Geometry: final body of the model. Coordinates: model frame, mm. A direction names the side the tool comes from. Round coordinates to 2 decimals unless told otherwise and drop trailing zeros. Write each loop counter-clockwise with the first axis right and the second up, starting at its lowest first coordinate (ties: lowest second). Pieces come first, ordered by that corner, then holes. Notation, with made-up numbers: M 12.25,-4.5 L 21.25,-4.5 A15 ccw 21.25,0.5 Z; hole C 75,8.25 d1. An arc over 180 degrees is marked long. Answer as CSV lines item,"result". Start each with the question number.
Q1. Section query B-B on y = 0. Output: boundary loops of the cut face in (x, z).
Q2. Reachability of faces 1 (the flat face through (-1, 1, -7.914)), 2 (the flat face through (12, 28.5, -3.914)) from +Z, -Z, +X, -X, +Y, -Y: full face, straight path, thin tool, end or side. Return the list, or none.
Q3. Ray query, probe 1 along Y at (x, z) = (7, 17); probe 2 along Z at (x, y) = (31, -8); probe 3 along Z at (x, y) = (9, -32). Return the intervals inside material, ascending.
Q4. First-contact query: pin 1 (3 mm diameter, centred on x = 13.5, y = -9, fed in from +Z); pin 2 (1 mm diameter, centred on y = -5, z = 25, fed in from -X). Flat tips, straight axial feed; report the tip coordinate or a pass-through.
Q5. Mould query, pull axis Y, two halves, no side actions, for faces 3 (the cylindrical face through (-1.18, -36.836, -7.407)), 4 (the cylindrical face through (3.503, 0.154, 39.907)), 5 (the flat face through (10, -3, 89.086)). Classes: pulls with the +Y half, pulls with the -Y half, needs draft (parallel to the pull), parting line crosses it, or undercut.
Q6. Section query A-A on x = 7. Output: boundary loops of the cut face in (y, z), and give its area (3 significant figures).
Q7. Section query C-C on z = 10. Output: boundary loops of the cut face in (x, y), and give its area (3 significant figures).
```python
from build123d import *

# Parameters (mm, degrees)
FILLET_R = 3


with BuildPart() as part:
    # Sketch → Revolution (revolve)
    with BuildSketch(Plane(origin=(7, 0, 0), x_dir=(1, 0, 0), z_dir=(0, -1, 0))):
        Polygon((37.732979, -7.91416), (37.732979, -3.91416), (28.608906, -3.91416), (28.608906, 0.08584), (21.351952, 0.08584), (21.351952, 4.08584), (6, 4.08584), (6, 89.08584), (3.5, 89.08584), (3.5, -7.91416), align=None)
    revolve(axis=Axis((7, 0, 0), (0, 0, 1)))

    # Fillet
    fillet_edges = [part.edges().sort_by_distance(p)[0] for p in [
        (-14.351952, 0, 4.08584),
        (-21.608906, 0, 0.08584),
        (-30.732979, 0, -3.91416),
    ]]
    fillet(fillet_edges, radius=FILLET_R)


solid = part.part
```
Entries:
1,outline,"M -30.73,-7.91 L 3.5,-7.91 L 3.5,89.09 L 1,89.09 L 1,4.09 L -11.35,4.09 A3 ccw -14.35,1.09 L -14.35,0.09 L -18.61,0.09 A3 ccw -21.61,-2.91 L -21.61,-3.91 L -27.73,-3.91 A3 ccw -30.73,-6.91 Z; M 10.5,-7.91 L 44.73,-7.91 L 44.73,-6.91 A3 ccw 41.73,-3.91 L 35.61,-3.91 L 35.61,-2.91 A3 ccw 32.61,0.09 L 28.35,0.09 L 28.35,1.09 A3 ccw 25.35,4.09 L 13,4.09 L 13,89.09 L 10.5,89.09 Z"
2,face 1,"-Z, +X, -X, +Y, -Y"
2,face 2,"+Z"
3,probe 1,"y = -6 to -3.5, 3.5 to 6"
3,probe 2,"z = -7.91 to 0.09"
3,probe 3,"z = -7.91 to -3.91"
4,pin 1,"stops at z = 4.09"
4,pin 2,"stops at x = 3.03"
5,face 3,"parting line crosses it"
5,face 4,"undercut"
5,face 5,"needs draft"
6,outline,"M -37.73,-7.91 L -3.5,-7.91 L -3.5,89.09 L -6,89.09 L -6,4.09 L -18.35,4.09 A3 ccw -21.35,1.09 L -21.35,0.09 L -25.61,0.09 A3 ccw -28.61,-2.91 L -28.61,-3.91 L -34.73,-3.91 A3 ccw -37.73,-6.91 Z; M 3.5,-7.91 L 37.73,-7.91 L 37.73,-6.91 A3 ccw 34.73,-3.91 L 28.61,-3.91 L 28.61,-2.91 A3 ccw 25.61,0.09 L 21.35,0.09 L 21.35,1.09 A3 ccw 18.35,4.09 L 6,4.09 L 6,89.09 L 3.5,89.09 Z"
6,area,"1,030 mm^2"
7,outline,"C 7,0 d12; hole C 7,0 d7"
7,area,"74.6 mm^2"
